from build123d import *

# Parameters (mm, degrees)
SKETCH1_R           = 2.0788
BOSS_EXTRUDE1_DEPTH = 70
SKETCH2_R           = 2
CUT_EXTRUDE1_DEPTH  = 15
SKETCH3_R           = 2
CUT_EXTRUDE2_DEPTH  = 15
CUT_EXTRUDE3_DEPTH  = 5
CUT_EXTRUDE4_DEPTH  = 5
CUT_EXTRUDE5_START  = -5
CUT_EXTRUDE5_DEPTH  = 5
FILLET1_R           = 2
SKETCH8_W           = 42.920227698
SKETCH8_H           = 32.849947737
CUT_EXTRUDE6_DEPTH  = 48


with BuildPart() as part:
    # Sketch1 → Boss-Extrude1 (new body)
    with BuildSketch(Plane(origin=(0, 0, 0), x_dir=(1, 0, 0), z_dir=(0, 1, 0))):
        with BuildLine():
            Line((-18.495, 5.34), (-9.495, 17.34))
            Line((-9.495, 17.34), (2.725, 8.175))
            Line((2.725, 8.175), (18, 8.175))
            Line((18, 8.175), (18, -6.825))
            Line((18, -6.825), (3, -6.825))
            Line((3, -6.825), (3, -10))
            Line((3, -10), (0, -10))
            ThreePointArc((0, -10), (-3.16227766, -9.486832981), (-6, -8))
            Line((-6, -8), (-8.4, -6.2))
            Line((-8.4, -6.2), (-6.495, -3.66))
            Line((-6.495, -3.66), (-18.495, 5.34))
        make_face()
        with Locations(Location((0, 0, 0), (0, 0, 270))):
            Circle(SKETCH1_R, mode=Mode.SUBTRACT)
    extrude(amount=BOSS_EXTRUDE1_DEPTH)

    # Sketch2 → Cut-Extrude1 (cut)
    with BuildSketch(Plane.XY.offset(6.825)):
        with Locations((10.5, 15)):
            Circle(SKETCH2_R)
        with Locations((10.5, 55)):
            Circle(SKETCH2_R)
    extrude(amount=-CUT_EXTRUDE1_DEPTH, mode=Mode.SUBTRACT)

    # Sketch3 → Cut-Extrude2 (cut)
    with BuildSketch(Plane(origin=(-4.095, 0, 5.46), x_dir=(0.8000000000000002, 0, 0.5999999999999999), z_dir=(-0.5999999999999999, 0, 0.8000000000000003))):
        with Locations((-10.5, 15)):
            Circle(SKETCH3_R)
        with Locations((-10.5, 55)):
            Circle(SKETCH3_R)
    extrude(amount=-CUT_EXTRUDE2_DEPTH, mode=Mode.SUBTRACT)

    # Sketch4 → Cut-Extrude3 (cut)
    with BuildSketch(Plane(origin=(4.905, 0, -6.54), x_dir=(-0.8000000000000002, 0, -0.5999999999999998), z_dir=(0.5999999999999998, 0, -0.8000000000000002))):
        Polygon((10.5, 59.871392896), (6.28125, 57.435696448), (6.28125, 52.564303552), (10.5, 50.128607104), (14.71875, 52.564303552), (14.71875, 57.435696448), align=None)
        Polygon((10.5, 10.128607104), (14.71875, 12.564303552), (14.71875, 17.435696448), (10.5, 19.871392896), (6.28125, 17.435696448), (6.28125, 12.564303552), align=None)
    extrude(amount=-CUT_EXTRUDE3_DEPTH, mode=Mode.SUBTRACT)

    # Sketch5 → Cut-Extrude4 (cut)
    with BuildSketch(Plane(origin=(0, 0, -8.175), x_dir=(-1, 0, 0), z_dir=(0, 0, -1))):
        Polygon((-10.5, 50.128607104), (-6.28125, 52.564303552), (-6.28125, 57.435696448), (-10.5, 59.871392896), (-14.71875, 57.435696448), (-14.71875, 52.564303552), align=None)
        Polygon((-10.5, 10.128607104), (-6.28125, 12.564303552), (-6.28125, 17.435696448), (-10.5, 19.871392896), (-14.71875, 17.435696448), (-14.71875, 12.564303552), align=None)
    extrude(amount=-CUT_EXTRUDE4_DEPTH, mode=Mode.SUBTRACT)

    # Sketch7 → Cut-Extrude5 (cut)
    with BuildSketch(Plane(origin=(0, 70, 0), x_dir=(1, 0, 0), z_dir=(0, 1, 0)).offset(CUT_EXTRUDE5_START)):
        Polygon((-4.773906582, -0.97690802), (-0.83361646, 10.843962345), (2.725, 8.175), (7.173270575, 8.175), (3.232980454, -3.645870365), (-1.540926128, -4.622778385), align=None)
    extrude(amount=-CUT_EXTRUDE5_DEPTH, mode=Mode.SUBTRACT)

    # Fillet1
    fillet1_edges = [part.edges().sort_by_distance(p)[0] for p in [
        (2.725, 30, -8.175),
        (-18.495, 35, -5.34),
        (-9.495, 35, -17.34),
        (2.725, 67.5, -8.175),
        (18, 35, -8.175),
        (18, 35, 6.825),
    ]]
    fillet(fillet1_edges, radius=FILLET1_R)

    # Sketch8 → Cut-Extrude6 (cut)
    with BuildSketch(Plane.XZ):
        with Locations((0.986015294, -3.374502162)):
            Rectangle(SKETCH8_W, SKETCH8_H)
    extrude(amount=-CUT_EXTRUDE6_DEPTH, mode=Mode.SUBTRACT)


solid = part.part
Geometry: final body of the model. Coordinates: model frame, mm. A direction names the side the tool comes from. Give positions to 0.01 mm unless a question says otherwise; leave off trailing zeros. Loops run counter-clockwise (first coordinate to the right, second up) from the corner with the lowest first, then second, coordinate; pieces in that order, holes last. Notation, with made-up numbers: M 48.5,-27.75 L 73.5,-27.75 A21 cw 73.5,10.25 Z; hole C -35,-23 d4. An arc over 180 degrees is marked long. Put each result on its own line as item: value.
1) Cut plane B-B, the plane y = 64.25. Return the cut outline in (x, z) (3 decimals).
Computed values:
outline: M -17.295,-6.94 L -10.695,-15.74 A2 ccw -7.895,-16.14 L -0.834,-10.844 L -4.774,0.977 L -1.541,4.623 L 3.233,3.646 L 7.173,-8.175 L 16,-8.175 A2 ccw 18,-6.175 L 18,4.825 A2 ccw 16,6.825 L 3,6.825 L 3,10 L 0,10 A10 ccw -6,8 L -8.4,6.2 L -6.495,3.66 L -16.895,-4.14 A2 ccw Z
2) Cut plane A-A, the plane y = 53.75. Give the number of separate pieces and of enclosed holes in the cut face, plus the area to 3 significant figures.
Computed values:
separate pieces: 3
enclosed holes: 1
area: 405 mm^2
3) Reachability of faces 4 (the flat face through (10, 61, -8.175)), 5 (the flat face through (8.361, 58.636, -5.71)), 6 (the flat face through (-11.622, 58.846, -0.185)) from +Z, -Z, +X, -X, +Y, -Y: full face, straight path, thin tool, end or side. Return the list, or none.
Computed values:
face 4: -Z, +X, +Y, -Y
face 5: -Z
face 6: -X, +Y, -Y
4) Cut plane C-C, the plane x = 14. Return the cut outline in (y, z) (3 decimals), plus the area to 3 significant figures.
Computed values:
outline: M 48,-8.175 L 52.149,-8.175 L 52.149,-3.175 L 57.851,-3.175 L 57.851,-8.175 L 70,-8.175 L 70,6.825 L 48,6.825 Z
area: 301 mm^2
5) Mould query, pull axis Z, two halves, no side actions, for faces 1 (the flat face through (-3.31, 58.67, -9.62)), 2 (the cylindrical face through (-3.12, 58.85, 9.5)), 3 (the flat face through (12.43, 53.99, -3.175)). Classes: released by +Z, released by -Z, zero draft, split by the parting line, or undercut.
Computed values:
face 1: undercut
face 2: released by +Z
face 3: released by -Z
6) First-contact query: P1, Ø4, axis at x = 12, y = 56.5, coming from the -Z side (3 decimals); P2, Ø4, axis at y = 59.5, z = -13.5, coming from the +X side; P3, Ø1.5, axis at x = -1, y = 58, coming from the +Z side. Flat tips, straight axial feed; report the tip coordinate or a pass-through.
Computed values:
P1: stops at z = -3.175
P2: stops at x = -1.71
P3: stops at z = 10
7) Material intervals for L1, parallel to Y at x = 1.5, z = -7.75; L2, parallel to Y at x = 10.5, z = -0.5; L3, parallel to Z at x = 8, y = 67.5 (3 decimals), sorted ascending. Write a range as from..to.
Computed values:
L1: y = 48..60, 65..70
L2: y = 48..53, 57..70
L3: z = -8.175..6.825
